Part model, mm, in its own coordinate system. Coordinates: 2 decimals unless noted, no trailing zeros. Write each loop counter-clockwise with the first axis right and the second up, starting at its lowest first coordinate (ties: lowest second). Pieces come first, ordered by that corner, then holes. Notation, with made-up numbers: M 88.25,64.25 L 115.25,64.25 A23 ccw 115.25,96.25 Z; hole C 6.25,39 d6. An arc over 180 degrees is marked long. Use a Markdown table: item, result. Add a question column.
Q1. Wall check: L1, parallel to X at y = -102, z = 2.7; L2, parallel to X at y = -121, z = 1.2; L3, parallel to Y at x = 134, z = 1.65. Give the ranges that are in metal, low to high. Write a range as from..to.
Q2. Slice it at B-B on x = 147. Write the cut outline in (y, z).
Q3. Slice it at C-C on z = 1.15. Count the separate pieces of the cut face and the enclosed holes in it, then the cut area to 3 significant figures.
Q4. Slice it at D-D on y = -101. Write the cut outline in (x, z), then the cut area to 3 significant figures.
Q5. Slice it at A-A on y = -78. Write the cut outline in (x, z).
Q6. Mould opens along Y. For faces 1 (the flat face through (131, -120, 3)), 2 (the cylindrical face through (113.377, -81.765, 1.479)), 3 (the flat face through (137, -71.866, 1)) say: released by +Y, released by -Y, zero draft, split by the parting line, or undercut.
from build123d import *

# Parameters (mm, degrees)
SKETCH1_R           = 2.3
SKETCH1_R_2         = 1.737885662
SKETCH1_R_3         = 1.873200063
SKETCH1_R_4         = 1.722278718
SKETCH1_R_5         = 1.754205974
SKETCH1_R_6         = 15.469551166
SKETCH1_R_7         = 5
BOSS_EXTRUDE1_DEPTH = 3


with BuildPart() as part:
    # Sketch1 → Boss-Extrude1 (new body)
    with BuildSketch(Plane.XY):
        with BuildLine():
            Line((116.525823666, -71.866196008), (157.960700719, -71.866196008))
            ThreePointArc((157.960700719, -71.866196008), (165.031768531, -74.795128196), (167.960700719, -81.866196008))
            Line((167.960700719, -81.866196008), (167.960700719, -141.896756479))
            ThreePointArc((167.960700719, -141.896756479), (165.031768531, -148.967824291), (157.960700719, -151.896756479))
            Line((157.960700719, -151.896756479), (116.525823666, -151.896756479))
            ThreePointArc((116.525823666, -151.896756479), (109.454755854, -148.967824291), (106.525823666, -141.896756479))
            Line((106.525823666, -141.896756479), (106.525823666, -81.866196008))
            ThreePointArc((106.525823666, -81.866196008), (109.454755854, -74.795128196), (116.525823666, -71.866196008))
        make_face()
        with Locations((115.674612816, -101.866196008)):
            Circle(SKETCH1_R, mode=Mode.SUBTRACT)
        with Locations((115.674612816, -121.866196008)):
            Circle(SKETCH1_R, mode=Mode.SUBTRACT)
        with Locations((135.674612816, -141.866196008)):
            Circle(SKETCH1_R, mode=Mode.SUBTRACT)
        with Locations((135.674612816, -81.866196008)):
            Circle(SKETCH1_R, mode=Mode.SUBTRACT)
        with Locations((115.674612816, -81.866196008)):
            Circle(SKETCH1_R, mode=Mode.SUBTRACT)
        with Locations((115.674612816, -141.866196008)):
            Circle(SKETCH1_R, mode=Mode.SUBTRACT)
        with Locations((130.460700719, -96.091712302)):
            Circle(SKETCH1_R_2, mode=Mode.SUBTRACT)
        with Locations((161.460700719, -96.091712302)):
            Circle(SKETCH1_R_3, mode=Mode.SUBTRACT)
        with Locations((130.460700719, -127.091712302)):
            Circle(SKETCH1_R_4, mode=Mode.SUBTRACT)
        with Locations((161.460700719, -127.091712302)):
            Circle(SKETCH1_R_5, mode=Mode.SUBTRACT)
        with Locations((145.960700719, -111.591712302)):
            Circle(SKETCH1_R_6, mode=Mode.SUBTRACT)
        with Locations((157.960700719, -81.591712302)):
            Circle(SKETCH1_R_7, mode=Mode.SUBTRACT)
        with Locations((157.960700719, -141.591712302)):
            Circle(SKETCH1_R_7, mode=Mode.SUBTRACT)
    extrude(amount=BOSS_EXTRUDE1_DEPTH)


solid = part.part
Recorded:
| question | item | result |
|---|---|---|
| 1 | L1 | 106.53..113.38, 117.97..133.82, 158.1..167.96 |
| 1 | L2 | 106.53..113.54, 117.81..133.68, 158.24..167.96 |
| 1 | L3 | -151.9..-143.44, -140.29..-121.4, -101.78..-83.44, -80.29..-71.87 |
| 2 | outline | M -151.9,0 L -127.03,0 L -127.03,3 L -151.9,3 Z; M -96.16,0 L -71.87,0 L -71.87,3 L -96.16,3 Z |
| 3 | separate pieces | 1 |
| 3 | enclosed holes | 13 |
| 3 | area | 3,780 mm² |
| 4 | outline | M 106.53,0 L 113.54,0 L 113.54,3 L 106.53,3 Z; M 117.81,0 L 134.69,0 L 134.69,3 L 117.81,3 Z; M 157.24,0 L 167.96,0 L 167.96,3 L 157.24,3 Z |
| 4 | area | 104 mm² |
| 5 | outline | M 107.3,0 L 154.48,0 L 154.48,3 L 107.3,3 Z; M 161.44,0 L 167.18,0 L 167.18,3 L 161.44,3 Z |
| 6 | face 1 | zero draft |
| 6 | face 2 | undercut |
| 6 | face 3 | released by +Y |
